CAD build for the part. Positions are in the model's coordinates, mm. Face numbers are marked on the shaded views. A direction names the side the tool comes from. Coordinates: 2 decimals unless noted, no trailing zeros. Write each loop counter-clockwise with the first axis right and the second up, starting at its lowest first coordinate (ties: lowest second). Pieces come first, ordered by that corner, then holes. Notation, with made-up numbers: (74.5, 15) -> (87.5, 15) arc R29 ccw to (87.5, 48) -> close; hole circle Ø7 at (48, 19.25). An arc over 180 degrees is marked (long way). Answer as CSV lines item,"result".
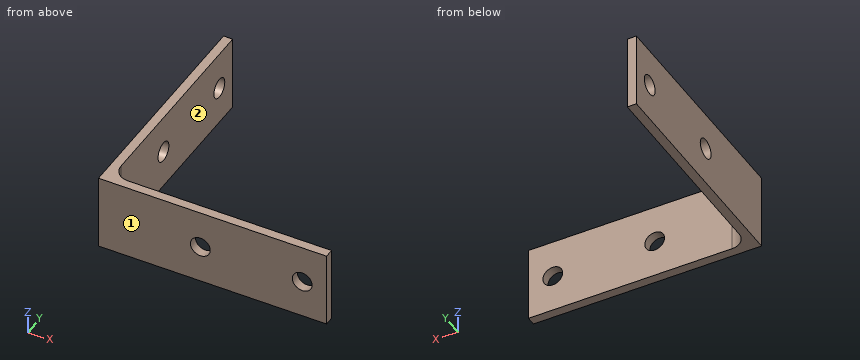
```python
from build123d import *

# Parameters (mm, degrees)
BOSS_EXTRUDE1_DEPTH = 6.35
FILLET1_R           = 2.54
SKETCH2_R           = 1.651
CUT_EXTRUDE1_DEPTH  = 54.195265541
SKETCH3_R           = 1.651
CUT_EXTRUDE2_DEPTH  = 54.195265541


with BuildPart() as part:
    # Sketch1 → Boss-Extrude1 (new, symmetric)
    with BuildSketch(Plane.XY):
        Polygon((0, 0), (38.1, 0), (38.1, 1.524), (36.576, 1.524), (1.524, 1.524), (1.524, 36.576), (1.524, 38.1), (0, 38.1), align=None)
    extrude(amount=BOSS_EXTRUDE1_DEPTH, both=True)

    # Fillet1
    fillet1_edges = [part.edges().sort_by_distance(p)[0] for p in [
        (1.524, 1.524, 0),
    ]]
    fillet(fillet1_edges, radius=FILLET1_R)

    # Sketch2 → Cut-Extrude1 (cut, through all)
    with BuildSketch(Plane(origin=(1.524, 0, 0), x_dir=(0, 0, -1), z_dir=(1, 0, 0))):
        with Locations(Location((0, 34.036, 0), (0, 0, 90))):
            Circle(SKETCH2_R)
        with Locations(Location((0, 17.018, 0), (0, 0, 90))):
            Circle(SKETCH2_R)
    extrude(amount=-CUT_EXTRUDE1_DEPTH, mode=Mode.SUBTRACT)

    # Sketch3 → Cut-Extrude2 (cut, through all)
    with BuildSketch(Plane(origin=(0, 1.524, 0), x_dir=(1, 0, 0), z_dir=(0, 1, 0))):
        with Locations(Location((17.018, 0, 0), (0, 0, 270))):
            Circle(SKETCH3_R)
        with Locations(Location((34.036, 0, 0), (0, 0, 270))):
            Circle(SKETCH3_R)
    extrude(amount=-CUT_EXTRUDE2_DEPTH, mode=Mode.SUBTRACT)


solid = part.part
```
Item 1: Saw through at D-D on y = 5.5. Give the cut face in (x, z), and give its area (3 significant figures).
Answer below:
outline,"(0, -6.35) -> (1.52, -6.35) -> (1.52, 6.35) -> (0, 6.35) -> close"
area,"19.4 mm2"
Item 2: Wall check: line 1 (X direction, y = 0.8, z = 0) (3 decimals); line 2 (X direction, y = 9, z = -2.75). Give the ranges that are in metal, low to high. Write a range as from..to.
Answer below:
line 1,"x = 0..15.367, 18.669..32.385, 35.687..38.1"
line 2,"x = 0..1.52"
Item 3: Flat gauge pins, fed straight in: pin 1 (1.5 mm diameter, centred on x = 15.5, z = 0, fed in from +Y); pin 2 (4 mm diameter, centred on y = 34.036, z = 0, fed in from +X); pin 3 (5 mm diameter, centred on x = 11, y = 5.5, fed in from -Z). Where does each tip first touch, or does it go through?
Answer below:
pin 1,"stops at y = 1.52"
pin 2,"stops at x = 1.52"
pin 3,"passes through"
Item 4: Saw through at B-B on x = 16. Give the cut face in (y, z).
Answer below:
outline,"(0, -6.35) -> (1.52, -6.35) -> (1.52, -1.3) -> (0, -1.3) -> close; (0, 1.3) -> (1.52, 1.3) -> (1.52, 6.35) -> (0, 6.35) -> close"
Item 5: Saw through at C-C on z = 2.75. Give the cut face in (x, y), and give its area (3 significant figures).
Answer below:
outline,"(0, 0) -> (38.1, 0) -> (38.1, 1.52) -> (4.06, 1.52) arc R2.54 cw to (1.52, 4.06) -> (1.52, 38.1) -> (0, 38.1) -> close"
area,"115 mm2"
Item 6: Saw through at A-A on z = 0. Give the cut face in (x, y) (3 decimals).
Answer below:
outline,"(0, 0) -> (15.367, 0) -> (15.367, 1.524) -> (4.064, 1.524) arc R2.54 cw to (1.524, 4.064) -> (1.524, 15.367) -> (0, 15.367) -> close; (0, 18.669) -> (1.524, 18.669) -> (1.524, 32.385) -> (0, 32.385) -> close; (0, 35.687) -> (1.524, 35.687) -> (1.524, 38.1) -> (0, 38.1) -> close; (18.669, 0) -> (32.385, 0) -> (32.385, 1.524) -> (18.669, 1.524) -> close; (35.687, 0) -> (38.1, 0) -> (38.1, 1.524) -> (35.687, 1.524) -> close"
Item 7: 3-axis set-ups, long thin cutter, end or side, ignore diameter. For the marked faces 1 and 2: which of +Z, -Z, +X, -X, +Y, -Y reach the whole face in a straight line?
Answer below:
face 1,"+Z, -Z, +X, -X, -Y"
face 2,"+Z, -Z, +X, +Y"
